The model under review builds one solid part; all positions refer to its coordinate system, in mm. A direction names the side the tool comes from. Coordinates: 2 decimals unless noted, no trailing zeros. Order: outer loops, then holes, each group sorted by start corner. A loop starts at its lowest first (then second) coordinate and runs counter-clockwise, first axis right, second up.
from build123d import *

# Parameters (mm, degrees)
F0_W           = 60
F0_H           = 37.5
F0_R           = 2.25
F0_R_2         = 15.1
F1_DEPTH       = 26
F3_D           = 5.3
F3_CBORE_D     = 10
F3_CBORE_DEPTH = 5
F4_T1_DEPTH    = 51.7168298797
F5_R           = 1


# Not quite as in the source:
# - a fillet or chamfer that OpenCascade refuses, or shapes differently, is made with other operations: its cross-section is extruded or revolved along the edge and cut away or added


with BuildPart() as f1:
    # F0 (on Front) → F1 (new body)
    with BuildSketch(Plane.XZ):
        with Locations((0, 1.25)):
            Rectangle(F0_W, F0_H)
        with Locations((-20.3874953738, -10.25)):
            Circle(F0_R, mode=Mode.SUBTRACT)
        with Locations((-3.5, -0.5)):
            Circle(F0_R_2, mode=Mode.SUBTRACT)
        with Locations((13.3874953738, -10.25)):
            Circle(F0_R, mode=Mode.SUBTRACT)
        with Locations((-20.3874953738, 9.25)):
            Circle(F0_R, mode=Mode.SUBTRACT)
        with Locations((13.3874953738, 9.25)):
            Circle(F0_R, mode=Mode.SUBTRACT)
    extrude(amount=-F1_DEPTH)

    # F3 (through all)
    with Locations(Plane.XY.offset(20)):
        with Locations((-23, 13), (23, 13)):
            CounterBoreHole(F3_D / 2, F3_CBORE_D / 2, F3_CBORE_DEPTH)

    # F4: chamfer of 5 on 2 edges, made by hand

    # F4_s2 → F4_t1 (cut)
    with BuildSketch(Plane.XZ.offset(-38.8584149398)):
        Polygon((-30, 15), (-25, 20), (-30, 20), align=None)
        Polygon((30, 15), (25, 20), (30, 20), align=None)
    extrude(amount=F4_T1_DEPTH, mode=Mode.SUBTRACT)

    # F5
    f5_edges = [f1.edges().sort_by_distance(p)[0] for p in [
        (-18.6, 0, -0.5),
    ]]
    fillet(f5_edges, radius=F5_R)


solid = f1.part
(1) Insertion check: pin 1 Ø3 at (x, y) = (-21.5, 15) entering from +Z. The pin has a flat end and moves straight along its axis. Give the tip position at first contact, or say it passes through.
(2) Consider section A-A (z = -0.5). Give the boundary of the cut face in (x, y).
(3) Consider section C-C (y = 13). Give the boundary of the cut face in (x, z).
(4) Tool access review of faces 1 (the face through (0, 13, 20)), 2 (the face through (25, 11, 15)): name each direction out of +Z, -Z, +X, -X, +Y, -Y from which nothing blocks a thin tool from reaching the whole face with its end or side.
(5) Wall thickness on line 1 (Z direction, x = -20.5, y = 3.75); line 2 (Y direction, x = 23, z = 17.7); line 3 (Z direction, x = -3, y = 7.5): over which ranges is each line inside the solid? List them lowest first.
(6) The part is to be moulded in two halves that separate along Z. For faces 3 (the face through (-18.241, 12.818, 9.926)), 4 (the face through (29, 13, 16)), 5 (the face through (13, 0, 2)), say which applies: +Z half, -Z half, draft (parallel to the pull), parting line (faces both ways), or undercut.
(7) Consider section B-B (x = -3.5). Give the boundary of the cut face in (y, z), then the cut area to 3 significant figures.
(8) Consider section D-D (y = 7.25). Give the boundary of the cut face in (x, z).
Findings:
1. pin 1: stops at z = 15
2. outline: (-30, 0) - (-19.6, 0) arc R1 ccw to (-18.6, 1) - (-18.6, 26) - (-30, 26) - close; (11.6, 1) arc R1 ccw to (12.6, 0) - (30, 0) - (30, 26) - (11.6, 26) - close; hole circle Ø5.3 at (-23, 13); hole circle Ø5.3 at (23, 13)
3. outline: (-30, -17.5) - (-25.65, -17.5) - (-25.65, 15) - (-28, 15) - (-28, 17) - (-30, 15) - close; (-20.35, -17.5) - (20.35, -17.5) - (20.35, 15) - (18, 15) - (18, 20) - (-18, 20) - (-18, 15) - (-20.35, 15) - (-20.35, 11.5) arc R2.25 cw to (-20.35, 7) - (-20.35, -8) arc R2.25 cw to (-20.35, -12.5) - close; (25.65, -17.5) - (30, -17.5) - (30, 15) - (28, 17) - (28, 15) - (25.65, 15) - close; hole circle Ø30.2 at (-3.5, -0.5); hole circle Ø4.5 at (13.39, -10.25); hole circle Ø4.5 at (13.39, 9.25)
4. face 1: +Z, +X, -X, +Y, -Y
4. face 2: +Z
5. line 1: z = -17.5 to -12.5, -8 to 7, 11.5 to 20
5. line 2: y = 0 to 8, 18 to 26
5. line 3: z = -17.5 to -15.59, 14.59 to 20
6. face 3: undercut
6. face 4: +Z half
6. face 5: draft
7. outline: (0, -17.5) - (26, -17.5) - (26, -15.6) - (1, -15.6) arc R1 ccw to (0, -16.6) - close; (0, 15.6) arc R1 ccw to (1, 14.6) - (26, 14.6) - (26, 20) - (0, 20) - close
7. area: 189 mm2
8. outline: (-30, -17.5) - (30, -17.5) - (30, 15) - (25, 20) - (-25, 20) - (-30, 15) - close; hole circle Ø4.5 at (-20.39, -10.25); hole circle Ø4.5 at (-20.39, 9.25); hole circle Ø30.2 at (-3.5, -0.5); hole circle Ø4.5 at (13.39, -10.25); hole circle Ø4.5 at (13.39, 9.25)
